```python
from build123d import *


with BuildPart() as part:
    # 草图1 → 旋转1 (revolve)
    with BuildSketch(Plane.XY, mode=Mode.PRIVATE) as revolve_1_sk:
        Polygon((0, 81.923883013), (6, 81.923883013), (6, 75.010759902), (9, 75.010759902), (9, 70.010759902), (7.57339192, 70.010759902), (7.57339192, 53.850491093), (9.5, 51.923883013), (9.5, -18.076116987), (0, -18.076116987), align=None)
    revolve(revolve_1_sk.sketch.rotate(Axis((0, 26.539226881, 0), (0, -1, 0)), 90), axis=Axis((0, 26.539226881, 0), (0, -1, 0)))

    # 草图2 → 旋转2 (revolve)
    with BuildSketch(Plane.XY, mode=Mode.PRIVATE) as revolve_2_sk:
        Polygon((7.5, -18.076116987), (7.5, -22.220066431), (9, -22.648998158), (9, -38.155089675), (5.305174294, -51.076116987), (5.305174294, -61.076116987), (3, -61.076116987), (3, -40.670715688), (0, -40.670715688), (0, -18.076116987), align=None)
    revolve(revolve_2_sk.sketch.rotate(Axis((0, -18.076116987, 0), (0, -1, 0)), 90), axis=Axis((0, -18.076116987, 0), (0, -1, 0)))


solid = part.part
```
Model file for the job. Use its own axes, mm. A direction names the side the tool comes from. Coordinates: 2 decimals unless noted, no trailing zeros. Order: outer loops, then holes, each group sorted by start corner. A loop starts at its lowest first (then second) coordinate and runs counter-clockwise, first axis right, second up. Notation, with made-up numbers: (64.5, 2) -> (93.5, 2) arc R26 ccw to (93.5, 31) -> close; hole circle Ø6 at (84.25, -3). An arc over 180 degrees is marked (long way). Return JSON: item names as keys, results as strings.
Item 1: Mould opens along X. For faces 1 (the face through (-6.083, -30.511, -6.633)), 2 (the face through (-0.9, -50.73, 2.86)), 3 (the face through (6, 75.011, -2)) say: pulls with the +X half, pulls with the -X half, needs draft (parallel to the pull), parting line crosses it, or undercut.
Model answer:
{"face 1": "parting line crosses it", "face 2": "undercut", "face 3": "needs draft"}
Item 2: 3-axis set-ups, long thin cutter, end or side, ignore diameter. For faces 4 (the face through (-1.802, 78.419, 5.723)), 5 (the face through (0, -40.671, 0)), 6 (the face through (6, 70.011, -5)): which of +Z, -Z, +X, -X, +Y, -Y reach the whole face in a straight line?
Model answer:
{"face 4": "+Y", "face 5": "-Y", "face 6": "none"}
Item 3: Pin check, flat tips, straight feed: P1, Ø1.5, axis at x = 6.5, y = 57, coming from the +Z side; P2, Ø4, axis at x = 6.5, y = -26.5, coming from the +Z side; P3, Ø5, axis at x = 0, z = 0, coming from the -Y side. Stop position of each tip, or through.
Model answer:
{"P1": "stops at z = 4.93", "P2": "stops at z = 7.79", "P3": "stops at y = -40.67"}
Item 4: Wall check: line 1 along X through (y, z) = (-56.25, 0); line 2 along X through (y, z) = (-50, 2.5); line 3 along X through (y, z) = (18, -0.5). Give the ranges that are in metal, low to high. Write a range as from..to.
Model answer:
{"line 1": "x = -5.31..-3, 3..5.31", "line 2": "x = -5.03..-1.66, 1.66..5.03", "line 3": "x = -9.49..9.49"}
Item 5: Slice it at C-C (y = 61.5). Write the cut outline in (x, z), then the cut area to 3 significant figures.
Model answer:
{"outline": "circle Ø15.15 at (0, 0)", "area": "180 mm²"}
Item 6: Slice it at D-D (y = 40). Write the cut outline in (x, z).
Model answer:
{"outline": "circle Ø19 at (0, 0)"}
